Input: part model. Units: mm. Frame: model coordinates. A direction names the side the tool comes from. Round coordinates to 2 decimals unless told otherwise and drop trailing zeros. Loops run counter-clockwise (first coordinate to the right, second up) from the corner with the lowest first, then second, coordinate; pieces in that order, holes last.
(1) Cut plane A-A, the plane x = 0. Output: boundary loops of the cut face in (y, z).
(2) Cut plane B-B, the plane y = 6. Output: boundary loops of the cut face in (x, z), and give its area (3 significant figures).
(3) Access query for faces 4 (the face through (9.23, 5.05, 2.54)), 5 (the face through (-4.513, 11.057, 0.891)), 6 (the face through (-3.4, 8, 3.4)), 7 (the face through (-4.51, 11.06, -0.9)). Directions: +Z, -Z, +X, -X, +Y, -Y. A direction counts if a zero-diameter tool reaches every point of the face in a straight line with its end or side. Return the directions, or none.
(4) Line query: line 1 (X direction, y = 6.5, z = 0); line 2 (X direction, y = 12.5, z = 0); line 3 (Y direction, x = 3, z = 3.5). Output: solid intervals per line, ascending.
(5) Draft query along Z for faces 1 (the face through (10, 4, 1.5)), 2 (the face through (-0.9, 11.06, 4.51)), 3 (the face through (0, 11.1, -4.2)). Return one class per face: released by +Z, released by -Z, zero draft, split by the parting line, or undercut.
(6) Cut plane D-D, the plane x = 8.25. Output: boundary loops of the cut face in (y, z).
(7) First-contact query: pin 1 Ø3 at (x, y) = (-2, 8) entering from -Z; pin 2 Ø1.9 at (x, y) = (10, 4) entering from -Z; pin 3 Ø4 at (x, y) = (7.5, 9) entering from +Z. Flat tips, straight axial feed; report the tip coordinate or a pass-through.
(8) Cut plane C-C, the plane z = 6.5. Output: boundary loops of the cut face in (x, y), and give its area (3 significant figures).
from build123d import *

# Parameters (mm, degrees)
SKETCH1_R           = 8
BOSS_EXTRUDE1_DEPTH = 8
SKETCH2_R           = 4.6
BOSS_EXTRUDE2_DEPTH = 6.2
CUT_EXTRUDE2_START  = -6.2
CUT_EXTRUDE2_DEPTH  = 6.2
SKETCH3_R           = 6
BOSS_EXTRUDE3_DEPTH = 1.4
CHAMFER1_SIZE       = 1.3
SKETCH4_R           = 2.75
BOSS_EXTRUDE4_DEPTH = 11
CUT_EXTRUDE1_DEPTH  = 2
SKETCH7_R           = 1.5
CUT_EXTRUDE3_DEPTH  = 21.696859757


with BuildPart() as part:
    # Sketch1 → Boss-Extrude1 (new body)
    with BuildSketch(Plane(origin=(0, 0, 0), x_dir=(1, 0, 0), z_dir=(0, 1, 0))):
        with Locations(Location((0, 0, 0), (0, 0, 270))):
            Circle(SKETCH1_R)
    extrude(amount=BOSS_EXTRUDE1_DEPTH)

    # Sketch2 → Boss-Extrude2 (add)
    with BuildSketch(Plane(origin=(0, 8, 0), x_dir=(1, 0, 0), z_dir=(0, 1, 0))):
        with Locations(Location((0, 0, 0), (0, 0, 90))):
            Circle(SKETCH2_R)
    extrude(amount=BOSS_EXTRUDE2_DEPTH)

    # Sketch6 → Cut-Extrude2 (cut)
    with BuildSketch(Plane(origin=(0, 14.2, 0), x_dir=(1, 0, 0), z_dir=(0, 1, 0)).offset(CUT_EXTRUDE2_START)):
        with BuildLine():
            Line((-0.450878846, 4.577849743), (-0.411671989, 4.179775852))
            ThreePointArc((-0.411671989, 4.179775852), (0, 4.2), (0.411671989, 4.179775852))
            Line((0.411671989, 4.179775852), (0.450878846, 4.577849743))
            ThreePointArc((0.450878846, 4.577849743), (0, 4.6), (-0.450878846, 4.577849743))
        make_face()
        with BuildLine():
            Line((2.168424989, 4.056837816), (1.979866295, 3.70406931))
            ThreePointArc((1.979866295, 3.70406931), (1.607270416, 3.880294037), (1.219195644, 4.01914941))
            Line((1.219195644, 4.01914941), (1.335309515, 4.401925544))
            ThreePointArc((1.335309515, 4.401925544), (1.760343789, 4.24984585), (2.168424989, 4.056837816))
        make_face()
        with BuildLine():
            Line((3.555848085, 2.918209107), (3.246643904, 2.664451793))
            ThreePointArc((3.246643904, 2.664451793), (2.969848481, 2.969848481), (2.664451793, 3.246643904))
            Line((2.664451793, 3.246643904), (2.918209107, 3.555848085))
            ThreePointArc((2.918209107, 3.555848085), (3.252691193, 3.252691193), (3.555848085, 2.918209107))
        make_face()
        with BuildLine():
            Line((4.401925544, 1.335309515), (4.01914941, 1.219195644))
            ThreePointArc((4.01914941, 1.219195644), (3.880294037, 1.607270416), (3.70406931, 1.979866295))
            Line((3.70406931, 1.979866295), (4.056837816, 2.168424989))
            ThreePointArc((4.056837816, 2.168424989), (4.24984585, 1.760343789), (4.401925544, 1.335309515))
        make_face()
        with BuildLine():
            Line((4.577849743, -0.450878846), (4.179775852, -0.411671989))
            ThreePointArc((4.179775852, -0.411671989), (4.2, 0), (4.179775852, 0.411671989))
            Line((4.179775852, 0.411671989), (4.577849743, 0.450878846))
            ThreePointArc((4.577849743, 0.450878846), (4.6, 0), (4.577849743, -0.450878846))
        make_face()
        with BuildLine():
            Line((4.056837816, -2.168424989), (3.70406931, -1.979866295))
            ThreePointArc((3.70406931, -1.979866295), (3.880294037, -1.607270416), (4.01914941, -1.219195644))
            Line((4.01914941, -1.219195644), (4.401925544, -1.335309515))
            ThreePointArc((4.401925544, -1.335309515), (4.24984585, -1.760343789), (4.056837816, -2.168424989))
        make_face()
        with BuildLine():
            Line((2.918209107, -3.555848085), (2.664451793, -3.246643904))
            ThreePointArc((2.664451793, -3.246643904), (2.969848481, -2.969848481), (3.246643904, -2.664451793))
            Line((3.246643904, -2.664451793), (3.555848085, -2.918209107))
            ThreePointArc((3.555848085, -2.918209107), (3.252691193, -3.252691193), (2.918209107, -3.555848085))
        make_face()
        with BuildLine():
            Line((1.335309515, -4.401925544), (1.219195644, -4.01914941))
            ThreePointArc((1.219195644, -4.01914941), (1.607270416, -3.880294037), (1.979866295, -3.70406931))
            Line((1.979866295, -3.70406931), (2.168424989, -4.056837816))
            ThreePointArc((2.168424989, -4.056837816), (1.760343789, -4.24984585), (1.335309515, -4.401925544))
        make_face()
        with BuildLine():
            Line((-0.450878846, -4.577849743), (-0.411671989, -4.179775852))
            ThreePointArc((-0.411671989, -4.179775852), (0, -4.2), (0.411671989, -4.179775852))
            Line((0.411671989, -4.179775852), (0.450878846, -4.577849743))
            ThreePointArc((0.450878846, -4.577849743), (0, -4.6), (-0.450878846, -4.577849743))
        make_face()
        with BuildLine():
            Line((-2.168424989, -4.056837816), (-1.979866295, -3.70406931))
            ThreePointArc((-1.979866295, -3.70406931), (-1.607270416, -3.880294037), (-1.219195644, -4.01914941))
            Line((-1.219195644, -4.01914941), (-1.335309515, -4.401925544))
            ThreePointArc((-1.335309515, -4.401925544), (-1.760343789, -4.24984585), (-2.168424989, -4.056837816))
        make_face()
        with BuildLine():
            Line((-3.555848085, -2.918209107), (-3.246643904, -2.664451793))
            ThreePointArc((-3.246643904, -2.664451793), (-2.969848481, -2.969848481), (-2.664451793, -3.246643904))
            Line((-2.664451793, -3.246643904), (-2.918209107, -3.555848085))
            ThreePointArc((-2.918209107, -3.555848085), (-3.252691193, -3.252691193), (-3.555848085, -2.918209107))
        make_face()
        with BuildLine():
            Line((-4.401925544, -1.335309515), (-4.01914941, -1.219195644))
            ThreePointArc((-4.01914941, -1.219195644), (-3.880294037, -1.607270416), (-3.70406931, -1.979866295))
            Line((-3.70406931, -1.979866295), (-4.056837816, -2.168424989))
            ThreePointArc((-4.056837816, -2.168424989), (-4.24984585, -1.760343789), (-4.401925544, -1.335309515))
        make_face()
        with BuildLine():
            Line((-4.577849743, 0.450878846), (-4.179775852, 0.411671989))
            ThreePointArc((-4.179775852, 0.411671989), (-4.2, 0), (-4.179775852, -0.411671989))
            Line((-4.179775852, -0.411671989), (-4.577849743, -0.450878846))
            ThreePointArc((-4.577849743, -0.450878846), (-4.6, 0), (-4.577849743, 0.450878846))
        make_face()
        with BuildLine():
            Line((-4.056837816, 2.168424989), (-3.70406931, 1.979866295))
            ThreePointArc((-3.70406931, 1.979866295), (-3.880294037, 1.607270416), (-4.01914941, 1.219195644))
            Line((-4.01914941, 1.219195644), (-4.401925544, 1.335309515))
            ThreePointArc((-4.401925544, 1.335309515), (-4.24984585, 1.760343789), (-4.056837816, 2.168424989))
        make_face()
        with BuildLine():
            Line((-2.918209107, 3.555848085), (-2.664451793, 3.246643904))
            ThreePointArc((-2.664451793, 3.246643904), (-2.969848481, 2.969848481), (-3.246643904, 2.664451793))
            Line((-3.246643904, 2.664451793), (-3.555848085, 2.918209107))
            ThreePointArc((-3.555848085, 2.918209107), (-3.252691193, 3.252691193), (-2.918209107, 3.555848085))
        make_face()
        with BuildLine():
            Line((-1.335309515, 4.401925544), (-1.219195644, 4.01914941))
            ThreePointArc((-1.219195644, 4.01914941), (-1.607270416, 3.880294037), (-1.979866295, 3.70406931))
            Line((-1.979866295, 3.70406931), (-2.168424989, 4.056837816))
            ThreePointArc((-2.168424989, 4.056837816), (-1.760343789, 4.24984585), (-1.335309515, 4.401925544))
        make_face()
    extrude(amount=CUT_EXTRUDE2_DEPTH, mode=Mode.SUBTRACT)

    # Sketch3 → Boss-Extrude3 (add)
    with BuildSketch(Plane(origin=(0, 14.2, 0), x_dir=(1, 0, 0), z_dir=(0, 1, 0))):
        with Locations(Location((0, 0, 0), (0, 0, 270))):
            Circle(SKETCH3_R)
    extrude(amount=BOSS_EXTRUDE3_DEPTH)

    # Chamfer1
    chamfer1_edges = [part.edges().sort_by_distance(p)[0] for p in [
        (0, 14.2, -6),
    ]]
    chamfer(chamfer1_edges, length=CHAMFER1_SIZE)

    # Sketch4 → Boss-Extrude4 (add)
    with BuildSketch(Plane(origin=(0, 0, 0), x_dir=(0, 0, -1), z_dir=(1, 0, 0))):
        with Locations(Location((0, 4, 0), (0, 0, 180))):
            Circle(SKETCH4_R)
    extrude(amount=BOSS_EXTRUDE4_DEPTH)

    # Sketch5 → Cut-Extrude1 (cut)
    with BuildSketch(Plane(origin=(11, 0, 0), x_dir=(0, 0, -1), z_dir=(1, 0, 0))):
        Polygon((0, 2.267949192), (1.5, 3.133974596), (1.5, 4.866025404), (0, 5.732050808), (-1.5, 4.866025404), (-1.5, 3.133974596), align=None)
    extrude(amount=-CUT_EXTRUDE1_DEPTH, mode=Mode.SUBTRACT)

    # Sketch7 → Cut-Extrude3 (cut, through all)
    with BuildSketch(Plane.XZ):
        with Locations(Location((0, 0, 0), (0, 0, 270))):
            Circle(SKETCH7_R)
    extrude(amount=-CUT_EXTRUDE3_DEPTH, mode=Mode.SUBTRACT)


solid = part.part
Reported:
1. outline: (0, -8) - (8, -8) - (8, -4.2) - (14.2, -4.2) - (14.2, -4.7) - (15.5, -6) - (15.6, -6) - (15.6, -1.5) - (0, -1.5) - close; (0, 1.5) - (15.6, 1.5) - (15.6, 6) - (15.5, 6) - (14.2, 4.7) - (14.2, 4.2) - (8, 4.2) - (8, 8) - (0, 8) - close
2. outline: (7.77, -1.89) - (11, -1.89) - (11, 1.89) - (7.77, 1.89) arc R8 ccw (long way) to start; hole circle Ø3 at (0, 0)
2. area: 206 mm2
3. face 4: +X
3. face 5: +Z, -X
3. face 6: none
3. face 7: -Z, -X
4. line 1: x = -8 to -1.5, 1.5 to 11
4. line 2: x = -4.2 to -1.5, 1.5 to 4.2
4. line 3: y = 0 to 8, 14.2 to 15.6
5. face 1: undercut
5. face 2: released by +Z
5. face 3: released by -Z
6. outline: circle Ø5.5 at (4, 0)
7. pin 1: stops at z = -7.98
7. pin 2: stops at z = -2.75
7. pin 3: stops at z = 5.54
8. outline: (-4.66, 0) - (4.66, 0) - (4.66, 8) - (-4.66, 8) - close
8. area: 74.6 mm2
